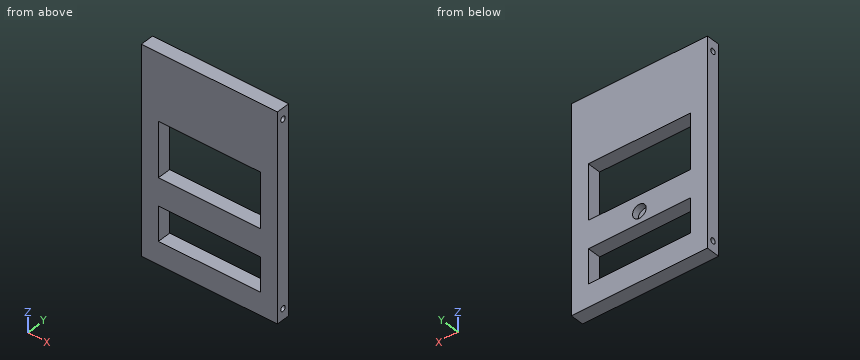
from build123d import *

# Parameters (mm, degrees)
SKETCH2_W           = 100
SKETCH2_H           = 150
BOSS_EXTRUDE1_DEPTH = 10
SKETCH3_R           = 5
MOUNTHOLE_DEPTH     = 5
SKETCH4_R           = 2
CUT_EXTRUDE2_DEPTH  = 101
SKETCH5_R           = 2
CUT_EXTRUDE3_DEPTH  = 101
SKETCH14_W          = 75
SKETCH14_H          = 25
SKETCH14_H_2        = 40
CUT_EXTRUDE7_DEPTH  = 11


with BuildPart() as part:
    # Sketch2 → Boss-Extrude1 (new body)
    with BuildSketch(Plane(origin=(0, 0, 0), x_dir=(1, 0, 0), z_dir=(0, 1, 0))):
        with Locations((50, 75)):
            Rectangle(SKETCH2_W, SKETCH2_H)
    extrude(amount=BOSS_EXTRUDE1_DEPTH)

    # Sketch3 → MountHole (cut)
    with BuildSketch(Plane(origin=(0, 10, 0), x_dir=(1, 0, 0), z_dir=(0, 1, 0))):
        with Locations((50, 100)):
            Circle(SKETCH3_R)
    extrude(amount=-MOUNTHOLE_DEPTH, mode=Mode.SUBTRACT)

    # Sketch4 → Cut-Extrude2 (cut, through all)
    with BuildSketch(Plane.ZY):
        with Locations((-8, 5)):
            Circle(SKETCH4_R)
    extrude(amount=-CUT_EXTRUDE2_DEPTH, mode=Mode.SUBTRACT)

    # Sketch5 → Cut-Extrude3 (cut, through all)
    with BuildSketch(Plane.ZY):
        with Locations((-142, 5)):
            Circle(SKETCH5_R)
    extrude(amount=-CUT_EXTRUDE3_DEPTH, mode=Mode.SUBTRACT)

    # Sketch14 → Cut-Extrude7 (cut, through all)
    with BuildSketch(Plane(origin=(0, 10, 0), x_dir=(1, 0, 0), z_dir=(0, 1, 0))):
        with Locations((50, 121)):
            Rectangle(SKETCH14_W, SKETCH14_H)
        with Locations((50, 68.5)):
            Rectangle(SKETCH14_W, SKETCH14_H_2)
    extrude(amount=-CUT_EXTRUDE7_DEPTH, mode=Mode.SUBTRACT)


solid = part.part
Could you check a few things on this model? Use its own coordinates, in mm. Give positions to 0.01 mm unless a question says otherwise; leave off trailing zeros. Order: outer loops, then holes, each group sorted by start corner. A loop starts at its lowest first (then second) coordinate and runs counter-clockwise, first axis right, second up. Notation, with made-up numbers: (-29, 19) -> (-2, 19) arc R23 cw to (-2, 56) -> close; hole circle Ø5 at (5, 74.5). An arc over 180 degrees is marked (long way). Return JSON: item names as keys, results as strings.
1. Imagine slicing it at B-B on z = -116.5. List the corners of the cut face in (x, y) for me.
Answer list:
{"outline": "(0, 0) -> (12.5, 0) -> (12.5, 10) -> (0, 10) -> close; (87.5, 0) -> (100, 0) -> (100, 10) -> (87.5, 10) -> close"}
2. I need wall thicknesses on line 1 (Z direction, x = 83.5, y = 9.5); line 2 (X direction, y = 7.25, z = -115); line 3 (Z direction, x = 50, y = 8.35). Which ranges of each line are inside material? Lowest first, please. Write a range as from..to.
Answer list:
{"line 1": "z = -150..-133.5, -108.5..-88.5, -48.5..0", "line 2": "x = 0..12.5, 87.5..100", "line 3": "z = -150..-133.5, -108.5..-105, -95..-88.5, -48.5..0"}
3. Imagine slicing it at C-C on x = 69. List the corners of the cut face in (y, z) for me, then the cut area to 3 significant figures.
Answer list:
{"outline": "(0, -150) -> (10, -150) -> (10, -133.5) -> (0, -133.5) -> close; (0, -108.5) -> (10, -108.5) -> (10, -88.5) -> (0, -88.5) -> close; (0, -48.5) -> (10, -48.5) -> (10, 0) -> (0, 0) -> close; hole circle Ø4 at (5, -142); hole circle Ø4 at (5, -8)", "area": "825 mm2"}
4. Imagine slicing it at D-D on z = -8. List the corners of the cut face in (x, y) for me.
Answer list:
{"outline": "(0, 0) -> (100, 0) -> (100, 3) -> (0, 3) -> close; (0, 7) -> (100, 7) -> (100, 10) -> (0, 10) -> close"}
5. Imagine slicing it at A-A on x = 50. List the corners of the cut face in (y, z) for me, then the cut area to 3 significant figures.
Answer list:
{"outline": "(0, -150) -> (10, -150) -> (10, -133.5) -> (0, -133.5) -> close; (0, -108.5) -> (10, -108.5) -> (10, -105) -> (5, -105) -> (5, -95) -> (10, -95) -> (10, -88.5) -> (0, -88.5) -> close; (0, -48.5) -> (10, -48.5) -> (10, 0) -> (0, 0) -> close; hole circle Ø4 at (5, -142); hole circle Ø4 at (5, -8)", "area": "775 mm2"}
